Check sheet for the modelled part. Datum: model origin and axes. Units: mm. Round coordinates to 2 decimals unless told otherwise and drop trailing zeros. Order: outer loops, then holes, each group sorted by start corner. A loop starts at its lowest first (then second) coordinate and runs counter-clockwise, first axis right, second up.
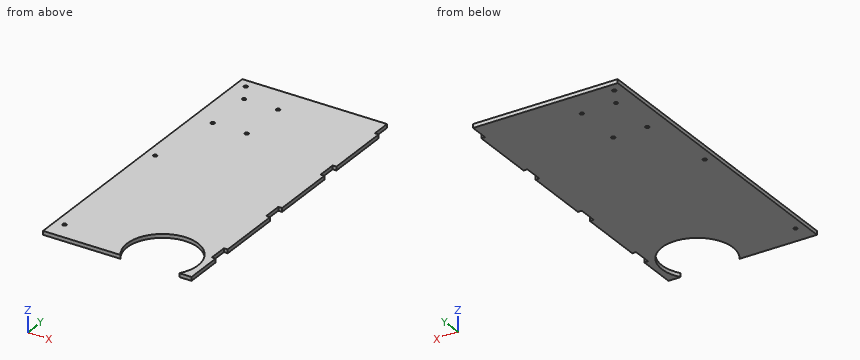
from build123d import *

# Parameters (mm, degrees)
SKETCH1_W           = 165
SKETCH1_H           = 330
BOSS_EXTRUDE1_DEPTH = 4
SKETCH2_R           = 37.5
CUT_EXTRUDE1_DEPTH  = 202.285866369
SKETCH4_W           = 8
SKETCH4_H           = 300
CUT_EXTRUDE3_DEPTH  = 202.285866369
SKETCH3_W           = 4
SKETCH3_H           = 20
CUT_EXTRUDE2_DEPTH  = 202.285866369
SKETCH5_W           = 8
SKETCH5_H           = 30
CUT_EXTRUDE4_DEPTH  = 202.285866369
SKETCH6_R           = 2
CUT_EXTRUDE5_DEPTH  = 198.838317825
SKETCH7_R           = 2
CUT_EXTRUDE6_DEPTH  = 198.838317825


with BuildPart() as part:
    # Sketch1 → Boss-Extrude1 (new body)
    with BuildSketch(Plane.XY):
        with Locations((7.5, -15)):
            Rectangle(SKETCH1_W, SKETCH1_H)
    extrude(amount=BOSS_EXTRUDE1_DEPTH)

    # Sketch2 → Cut-Extrude1 (cut, through all)
    with BuildSketch(Plane.XY.offset(4)):
        with Locations((38, -159)):
            Circle(SKETCH2_R)
    extrude(amount=-CUT_EXTRUDE1_DEPTH, mode=Mode.SUBTRACT)

    # Sketch4 → Cut-Extrude3 (cut, through all)
    with BuildSketch(Plane(origin=(0, 0, 0), x_dir=(-1, 0, 0), z_dir=(0, 0, -1))):
        with Locations((-86, 0)):
            Rectangle(SKETCH4_W, SKETCH4_H)
    extrude(amount=-CUT_EXTRUDE3_DEPTH, mode=Mode.SUBTRACT)

    # Sketch3 → Cut-Extrude2 (cut, through all)
    with BuildSketch(Plane(origin=(0, 0, 0), x_dir=(-1, 0, 0), z_dir=(0, 0, -1))):
        with Locations((-80, 140)):
            Rectangle(SKETCH3_W, SKETCH3_H)
        with Locations((-80, 50)):
            Rectangle(SKETCH3_W, SKETCH3_H)
        with Locations((-80, -40)):
            Rectangle(SKETCH3_W, SKETCH3_H)
        with Locations((-80, -130)):
            Rectangle(SKETCH3_W, SKETCH3_H)
    extrude(amount=-CUT_EXTRUDE2_DEPTH, mode=Mode.SUBTRACT)

    # Sketch5 → Cut-Extrude4 (cut, through all)
    with BuildSketch(Plane.XY.offset(4)):
        with Locations((86, -165)):
            Rectangle(SKETCH5_W, SKETCH5_H)
    extrude(amount=-CUT_EXTRUDE4_DEPTH, mode=Mode.SUBTRACT)

    # Sketch6 → Cut-Extrude5 (cut, through all)
    with BuildSketch(Plane(origin=(0, 0, 0), x_dir=(-1, 0, 0), z_dir=(0, 0, -1))):
        with Locations((18, 120)):
            Circle(SKETCH6_R)
        with Locations((54, 120)):
            Circle(SKETCH6_R)
        with Locations((18, 68)):
            Circle(SKETCH6_R)
        with Locations((54, 68)):
            Circle(SKETCH6_R)
    extrude(amount=-CUT_EXTRUDE5_DEPTH, mode=Mode.SUBTRACT)

    # Sketch7 → Cut-Extrude6 (cut, through all)
    with BuildSketch(Plane.XY.offset(4)):
        with Locations((-65, 140)):
            Circle(SKETCH7_R)
        with Locations((-65, -10)):
            Circle(SKETCH7_R)
        with Locations((-65, -160)):
            Circle(SKETCH7_R)
    extrude(amount=-CUT_EXTRUDE6_DEPTH, mode=Mode.SUBTRACT)


solid = part.part
1) Sectioned sample at B-B on x = 59.5. Record the cut outline in (y, z), and give its area (3 significant figures).
2) Gauge pin test, flat ends, axial feed: pin 1 (1.2 mm diameter, centred on y = -127.5, z = 3, fed in from +X); pin 2 (1.2 mm diameter, centred on x = 81, z = 2, fed in from +Y); pin 3 (2.5 mm diameter, centred on x = -65, y = -10, fed in from +Z); pin 4 (1 mm diameter, centred on x = 21.5, z = 1.5, fed in from -Y). Record the tip position at first contact, or that the pin passes through.
3) Scan lines: line 1 (Y direction, x = -65, z = 1.3); line 2 (X direction, y = -39.5, z = 1.2); line 3 (X direction, y = -142.5, z = 1.85). Record each from-to range of solid material in increasing order.
4) Sectioned sample at A-A on z = 0.95. Record the cut outline in (x, y).
Values found:
1. outline: (-128.28, 0) - (150, 0) - (150, 4) - (-128.28, 4) - close
1. area: 1,110 mm2
2. pin 1: stops at x = 78
2. pin 2: stops at y = 130
2. pin 3: passes through
2. pin 4: stops at y = -125.57
3. line 1: y = -180 to -162, -158 to -12, -8 to 138, 142 to 150
3. line 2: x = -75 to 78
3. line 3: x = -75 to 4.33, 71.67 to 82
4. outline: (-75, -180) - (6.93, -180) arc R37.5 cw (long way) to (69.07, -180) - (82, -180) - (82, -140) - (78, -140) - (78, -120) - (82, -120) - (82, -50) - (78, -50) - (78, -30) - (82, -30) - (82, 40) - (78, 40) - (78, 60) - (82, 60) - (82, 130) - (78, 130) - (78, 150) - (-75, 150) - close; hole circle Ø4 at (-65, -160); hole circle Ø4 at (-65, -10); hole circle Ø4 at (-65, 140); hole circle Ø4 at (-54, 68); hole circle Ø4 at (-54, 120); hole circle Ø4 at (-18, 68); hole circle Ø4 at (-18, 120)
